Geometry check sheet. Reference: drawing and pictorial views, mm from the part's lowest x, y, z. A direction names the side the tool comes from. Give positions to 0.01 mm unless a question says otherwise; leave off trailing zeros. Order: outer loops, then holes, each group sorted by start corner. A loop starts at its lowest first (then second) coordinate and runs counter-clockwise, first axis right, second up.
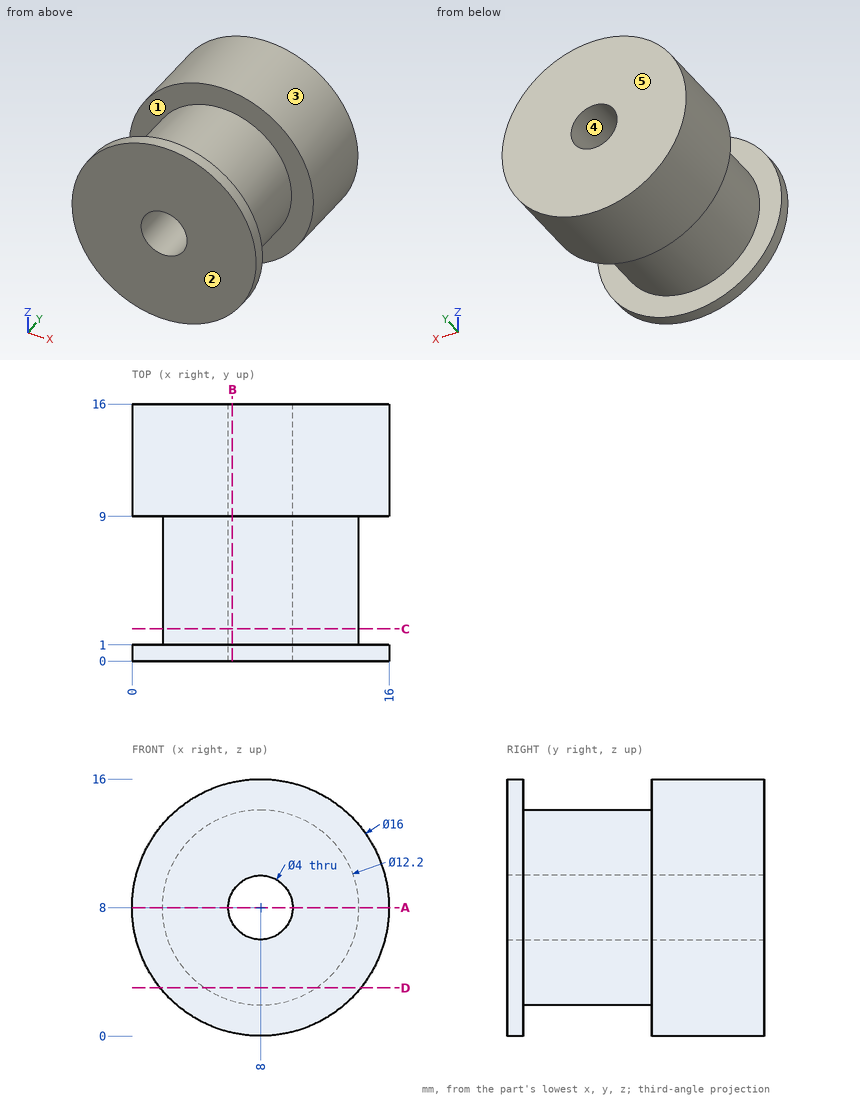
1) Depth check by flat-ended pin: pin 1 Ø5 at (y, z) = (2, 2) entering from -X; pin 2 Ø4 at (x, y) = (13.5, 13.5) entering from -Z; pin 3 Ø2 at (x, y) = (8.5, 6.5) entering from -Z. Enter the tip coordinate at first touch or a pass-through.
Recorded:
pin 1: stops at x = 0.91
pin 2: stops at z = 0.81
pin 3: stops at z = 1.9
2) Draft check along X on the marked faces 3, 4 and 5. Enter one of: +X half, -X half, draft (parallel to the pull), parting line (faces both ways), or undercut.
Recorded:
face 3: parting line
face 4: undercut
face 5: draft
3) Section check C-C, the plane y = 2. Record the cut outline in (x, z).
Recorded:
outline: circle Ø12.2 at (8, 8); hole circle Ø4 at (8, 8)
4) Section check A-A, the plane z = 8. Record the cut outline in (x, y).
Recorded:
outline: (0, 0) - (6, 0) - (6, 16) - (0, 16) - (0, 9) - (1.9, 9) - (1.9, 1) - (0, 1) - close; (10, 0) - (16, 0) - (16, 1) - (14.1, 1) - (14.1, 9) - (16, 9) - (16, 16) - (10, 16) - close
5) Material ranges on L1, parallel to X at y = 8.75, z = 8; L2, parallel to Y at x = 13.25, z = 4.25; L3, parallel to X at y = 12.75, z = 8, recorded low to high.
Recorded:
L1: x = 1.9 to 6, 10 to 14.1
L2: y = 0 to 1, 9 to 16
L3: x = 0 to 6, 10 to 16
6) Section check B-B, the plane x = 6.25. Record the cut outline in (y, z), then the cut area to 3 significant figures.
Recorded:
outline: (0, 0.19) - (1, 0.19) - (1, 2.16) - (9, 2.16) - (9, 0.19) - (16, 0.19) - (16, 7.03) - (0, 7.03) - close; (0, 8.97) - (16, 8.97) - (16, 15.81) - (9, 15.81) - (9, 13.84) - (1, 13.84) - (1, 15.81) - (0, 15.81) - close
area: 187 mm2
7) Set-up check for the marked faces 1 and 2: record each of +Z, -Z, +X, -X, +Y, -Y from which the full face is reachable in a straight line by a thin tool's end or side.
Recorded:
face 1: none
face 2: +Z, -Z, +X, -X, -Y
8) Section check D-D, the plane z = 3. Record the cut outline in (x, y) (3 decimals).
Recorded:
outline: (1.755, 0) - (14.245, 0) - (14.245, 1) - (11.494, 1) - (11.494, 9) - (14.245, 9) - (14.245, 16) - (1.755, 16) - (1.755, 9) - (4.506, 9) - (4.506, 1) - (1.755, 1) - close
